Geometry: final body of the model. Coordinates: model frame, mm. Round coordinates to 2 decimals unless told otherwise and drop trailing zeros. Write each loop counter-clockwise with the first axis right and the second up, starting at its lowest first coordinate (ties: lowest second). Pieces come first, ordered by that corner, then holes. Notation, with made-up numbers: M 51.5,-19.5 L 105.5,-19.5 A13 cw 105.5,-11.5 Z; hole C -4.75,-8.75 d3. An arc over 180 degrees is marked long. Use one line per item in the form item = value. Start each with the question number.
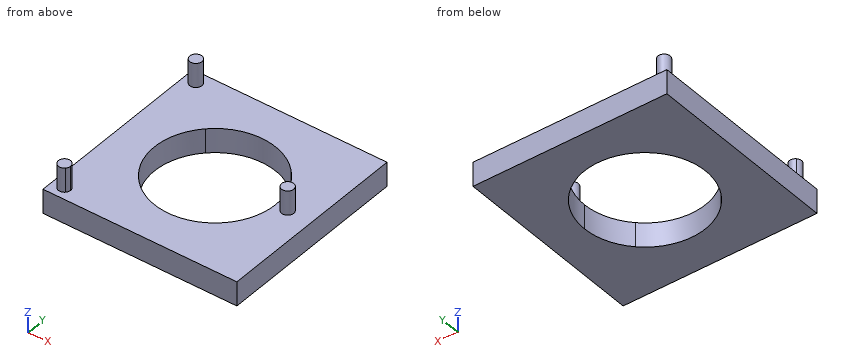
from build123d import *

# Parameters (mm, degrees)
F0_W     = 101.6
F0_H     = 101.6
F1_DEPTH = 12.7
F2_R     = 3.175
F3_DEPTH = 12.7
F4_R     = 3.175
F5_DEPTH = 12.7
F7_DEPTH = 25.4


with BuildPart() as f1:
    # F0 (on Top) → F1 (new body)
    with BuildSketch(Plane.XY):
        with Locations((-50.8, -50.8)):
            Rectangle(F0_W, F0_H)
    extrude(amount=F1_DEPTH)

    # F2 (on face) → F3 (join)
    with BuildSketch(Plane.XY.offset(12.7)):
        with BuildLine():
            Line((-95.25, -95.25), (-97.4950640303, -97.4950640303))
            ThreePointArc((-97.4950640303, -97.4950640303), (-95.25, -98.425), (-93.0049359697, -97.4950640303))
            Line((-93.0049359697, -97.4950640303), (-95.25, -95.25))
        make_face()
        with BuildLine():
            ThreePointArc((-93.0049359697, -93.0049359697), (-95.25, -92.075), (-97.4950640303, -93.0049359697))
            Line((-97.4950640303, -93.0049359697), (-95.25, -95.25))
            Line((-95.25, -95.25), (-93.0049359697, -93.0049359697))
        make_face()
        with BuildLine():
            Line((-95.25, -95.25), (-93.0049359697, -97.4950640303))
            ThreePointArc((-93.0049359697, -97.4950640303), (-92.3166824843, -96.4650198978), (-92.075, -95.25))
            ThreePointArc((-92.075, -95.25), (-92.3166824843, -94.0349801022), (-93.0049359697, -93.0049359697))
            Line((-93.0049359697, -93.0049359697), (-95.25, -95.25))
        make_face()
        with BuildLine():
            ThreePointArc((-97.4950640303, -93.0049359697), (-98.425, -95.25), (-97.4950640303, -97.4950640303))
            Line((-97.4950640303, -97.4950640303), (-95.25, -95.25))
            Line((-95.25, -95.25), (-97.4950640303, -93.0049359697))
        make_face()
        with Locations((-95.25, -6.35)):
            Circle(F2_R)
    extrude(amount=F3_DEPTH)

    # F4 (on face) → F5 (join)
    with BuildSketch(Plane.XY.offset(12.7)):
        with Locations((-12.7, -50.8)):
            Circle(F4_R)
    extrude(amount=F5_DEPTH)

    # F6 (on face) → F7 (cut)
    with BuildSketch(Plane.XY.offset(12.7)):
        with BuildLine():
            ThreePointArc((-73.2506403027, -28.3493596973), (-82.55, -50.8), (-73.2506403027, -73.2506403027))
            Line((-73.2506403027, -73.2506403027), (-50.8, -50.8))
            Line((-50.8, -50.8), (-73.2506403027, -28.3493596973))
        make_face()
        with BuildLine():
            Line((-50.8, -50.8), (-28.3493596973, -28.3493596973))
            ThreePointArc((-28.3493596973, -28.3493596973), (-50.8, -19.05), (-73.2506403027, -28.3493596973))
            Line((-73.2506403027, -28.3493596973), (-50.8, -50.8))
        make_face()
        with BuildLine():
            Line((-50.8, -50.8), (-28.3493596973, -73.2506403027))
            ThreePointArc((-28.3493596973, -73.2506403027), (-21.4668248428, -62.9501989776), (-19.05, -50.8))
            ThreePointArc((-19.05, -50.8), (-21.4668248428, -38.6498010224), (-28.3493596973, -28.3493596973))
            Line((-28.3493596973, -28.3493596973), (-50.8, -50.8))
        make_face()
        with BuildLine():
            ThreePointArc((-73.2506403027, -73.2506403027), (-50.8, -82.55), (-28.3493596973, -73.2506403027))
            Line((-28.3493596973, -73.2506403027), (-50.8, -50.8))
            Line((-50.8, -50.8), (-73.2506403027, -73.2506403027))
        make_face()
    extrude(amount=-F7_DEPTH, mode=Mode.SUBTRACT)


solid = f1.part
1. Section query B-B (x = -45.5). Return loops of the section in (y, z).
2. Ray query, probe 1 along Z at (x, y) = (-4, -17.5); probe 2 along X at (y, z) = (-93, 18); probe 3 along Y at (x, z) = (-64.5, 3). Return the intervals inside material, ascending.
3. Contact query for flat-ended pins moving along their axis: pin 1 (12 mm diameter, centred on x = -12.5, y = -58.5, fed in from -Z); pin 2 (2 mm diameter, centred on x = -91, y = -89.5, fed in from +Z); pin 3 (10 mm diameter, centred on y = -35, z = 18.5, fed in from +X). Output: stop coordinate, or through.
4. Section query A-A (z = 22.75). Return loops of the section in (x, y) (3 decimals).
5. Section query C-C (z = 2.5). Return loops of the section in (x, y), then the cut area to 3 significant figures.
6. Section query D-D (y = -37.5). Return loops of the section in (x, z).
Checks:
q1.outline = M -101.6,0 L -82.1,0 L -82.1,12.7 L -101.6,12.7 Z; M -19.5,0 L 0,0 L 0,12.7 L -19.5,12.7 Z
q2.probe_1 = 0 to 12.7
q2.probe_2 = -97.49 to -93.01
q2.probe_3 = -101.6 to -79.44, -22.16 to 0
q3.pin_1 = 0
q3.pin_2 = 12.7
q3.pin_3 = through
q4.outline = C -95.25,-95.25 d6.35; C -95.25,-6.35 d6.35; C -12.7,-50.8 d6.35
q5.outline = M -101.6,-101.6 L 0,-101.6 L 0,0 L -101.6,0 Z; hole C -50.8,-50.8 d63.5
q5.area = 7,160 mm^2
q6.outline = M -101.6,0 L -79.63,0 L -79.63,12.7 L -101.6,12.7 Z; M -21.97,0 L 0,0 L 0,12.7 L -21.97,12.7 Z
